Source: three-view drawing plus pictorial views. Frame: mm from the lowest corner of the part. Round coordinates to 2 decimals unless told otherwise and drop trailing zeros. Write each loop counter-clockwise with the first axis right and the second up, starting at its lowest first coordinate (ties: lowest second). Pieces come first, ordered by that corner, then holes. Notation, with made-up numbers: (75.5, 63.5) -> (99.5, 63.5) arc R30 cw to (99.5, 92.5) -> close; hole circle Ø8 at (10.25, 49). An arc over 180 degrees is marked (long way). Put each result on its own line as item: value.
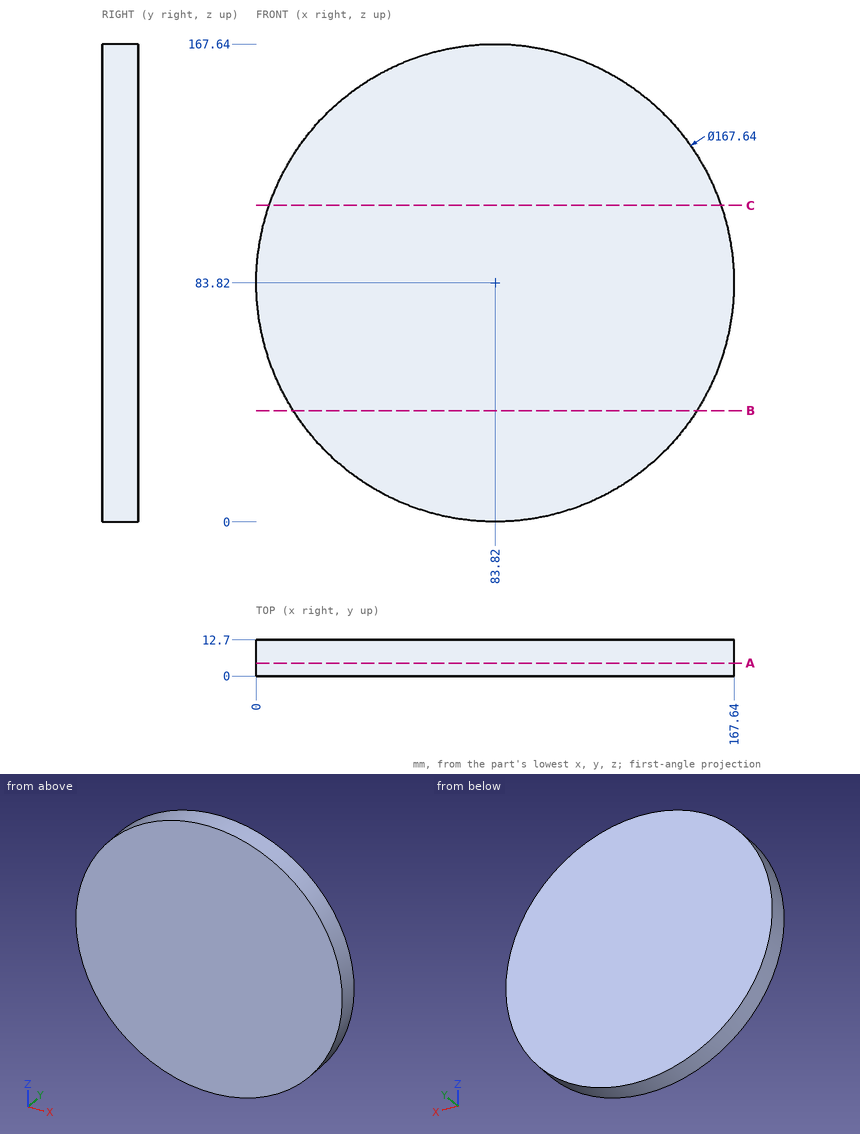
Q1. Cut plane B-B on z = 39. Output: boundary loops of the cut face in (x, y).
Ans:
outline: (12.99, 0) -> (154.65, 0) -> (154.65, 12.7) -> (12.99, 12.7) -> close
Q2. Material intervals for line 1 (Z direction, x = 85, y = 11.5); line 2 (Z direction, x = 106, y = 3.75); line 3 (X direction, y = 2.25, z = 11), sorted ascending. Write a range as [from, to].
Ans:
line 1: z = [0.01, 167.63]
line 2: z = [2.99, 164.65]
line 3: x = [42.31, 125.33]
Q3. Cut plane C-C on z = 111. Output: boundary loops of the cut face in (x, y).
Ans:
outline: (4.53, 0) -> (163.11, 0) -> (163.11, 12.7) -> (4.53, 12.7) -> close
Q4. Cut plane A-A on y = 4.5. Output: boundary loops of the cut face in (x, z).
Ans:
outline: circle Ø167.64 at (83.82, 83.82)
Q5. Pin query (flat end, axial travel): pin 1 (2 mm diameter, centred on x = 123.5, y = 4, fed in from -Z); pin 2 (4 mm diameter, centred on x = 128.5, y = 7.5, fed in from +Z); pin 3 (2 mm diameter, centred on x = 102, y = 6.5, fed in from -Z). Return the tip coordinate at first contact, or that it passes through.
Ans:
pin 1: stops at z = 9.46
pin 2: stops at z = 155.96
pin 3: stops at z = 1.78
